from build123d import *

# Parameters (mm, degrees)
SKETCH1_W           = 12
SKETCH1_H           = 12
BOSS_EXTRUDE1_DEPTH = 11
SHELL1_T            = -2
SKETCH3_R           = 0.625
CUT_EXTRUDE1_DEPTH  = 10
SKETCH4_W           = 12
SKETCH4_H           = 12
SKETCH4_W_2         = 11
SKETCH4_H_2         = 11
CUT_EXTRUDE2_DEPTH  = 12
SKETCH5_W           = 11
SKETCH5_H           = 11
CUT_EXTRUDE3_DEPTH  = 0.5


with BuildPart() as part:
    # Sketch1 → Boss-Extrude1 (new body)
    with BuildSketch(Plane(origin=(0, 0, 0), x_dir=(1, 0, 0), z_dir=(0, 1, 0))):
        with Locations((6, 6)):
            Rectangle(SKETCH1_W, SKETCH1_H)
    extrude(amount=BOSS_EXTRUDE1_DEPTH)

    # Shell1
    shell1_openings = [part.faces().sort_by_distance(p)[0] for p in [
        (6, 11, -6),
    ]]
    offset(amount=SHELL1_T, openings=shell1_openings, kind=Kind.INTERSECTION)

    # Sketch3 → Cut-Extrude1 (cut)
    with BuildSketch(Plane.XZ):
        with Locations((6, -4.73)):
            Circle(SKETCH3_R)
        with Locations((6, -7.27)):
            Circle(SKETCH3_R)
    extrude(amount=-CUT_EXTRUDE1_DEPTH, mode=Mode.SUBTRACT)

    # Sketch4 → Cut-Extrude2 (cut, through all)
    with BuildSketch(Plane(origin=(0, 11, 0), x_dir=(1, 0, 0), z_dir=(0, 1, 0))):
        with Locations((6, 6)):
            Rectangle(SKETCH4_W, SKETCH4_H)
        with Locations((6, 6)):
            Rectangle(SKETCH4_W_2, SKETCH4_H_2, mode=Mode.SUBTRACT)
    extrude(amount=-CUT_EXTRUDE2_DEPTH, mode=Mode.SUBTRACT)

    # Sketch5 → Cut-Extrude3 (cut)
    with BuildSketch(Plane.XZ):
        with Locations((6, -6)):
            Rectangle(SKETCH5_W, SKETCH5_H)
    extrude(amount=-CUT_EXTRUDE3_DEPTH, mode=Mode.SUBTRACT)


solid = part.part
Could you check a few things on this model? Use its own coordinates, in mm. A direction names the side the tool comes from. Coordinates: 2 decimals unless noted, no trailing zeros. Write each loop counter-clockwise with the first axis right and the second up, starting at its lowest first coordinate (ties: lowest second). Pieces come first, ordered by that corner, then holes. Notation, with made-up numbers: M 86.5,15 L 124.5,15 A25 cw 124.5,29 Z; hole C 46.25,-12 d6. An arc over 180 degrees is marked long. One line per question, with ' | ' between items.
1) For pin 1 Ø1.6 at (x, z) = (6, -4.73) entering from +Y; pin 2 Ø1.1 at (x, z) = (6, -7.27) entering from +Y, each with a flat end and sliding along its axis, tell me the tip position at first contact or that it passes through.
Checks:
pin 1: y = 2 | pin 2: through
2) Imagine slicing it at C-C, the plane z = -7.27. Write out the boundary of the cut face in (x, y) (3 decimals).
Checks:
outline: M 0.5,0.5 L 5.375,0.5 L 5.375,2 L 2,2 L 2,11 L 0.5,11 Z; M 6.625,0.5 L 11.5,0.5 L 11.5,11 L 10,11 L 10,2 L 6.625,2 Z
3) Imagine slicing it at D-D, the plane x = 9. Write out the boundary of the cut face in (y, z), and give its area (3 significant figures).
Checks:
outline: M 0.5,-11.5 L 11,-11.5 L 11,-10 L 2,-10 L 2,-2 L 11,-2 L 11,-0.5 L 0.5,-0.5 Z | area: 43.5 mm²
4) For faces 1 (the face through (5.92, 1.24, -6.65)), 2 (the face through (6, 6, -2)), which set-ups out of +Z, -Z, +X, -X, +Y, -Y let a thin tool reach every point of the face, with its end or its side?
Checks:
face 1: +Y, -Y | face 2: +Y
5) If we mould it in two halves opening along X, with no side actions, what happens to faces 3 (the face through (6, 6, -0.5)), 4 (the face through (0.5, 6, -6)), 5 (the face through (6, 2, -6))? For each: released by +X, released by -X, zero draft, split by the parting line, or undercut.
Checks:
face 3: zero draft | face 4: released by -X | face 5: undercut
6) Imagine slicing it at A-A, the plane y = 8.25. Write out the boundary of the cut face in (x, z), and give its area (3 significant figures).
Checks:
outline: M 0.5,-11.5 L 11.5,-11.5 L 11.5,-0.5 L 0.5,-0.5 Z; hole M 2,-10 L 10,-10 L 10,-2 L 2,-2 Z | area: 57.0 mm²
7) I need wall thicknesses on probe 1 along Z at (x, y) = (6, 1.35) (3 decimals); probe 2 along Z at (x, y) = (3.5, 9.75); probe 3 along X at (y, z) = (5, -6.5). Which ranges of each line are inside material? Lowest first, please. Write a range as [from, to].
Checks:
probe 1: [-11.5, -7.895], [-6.645, -5.355], [-4.105, -0.5] | probe 2: [-11.5, -10], [-2, -0.5] | probe 3: [0.5, 2], [10, 11.5]
8) Imagine slicing it at B-B, the plane x = 6. Write out the boundary of the cut face in (y, z) (3 decimals).
Checks:
outline: M 0.5,-11.5 L 11,-11.5 L 11,-10 L 2,-10 L 2,-7.895 L 0.5,-7.895 Z; M 0.5,-6.645 L 2,-6.645 L 2,-5.355 L 0.5,-5.355 Z; M 0.5,-4.105 L 2,-4.105 L 2,-2 L 11,-2 L 11,-0.5 L 0.5,-0.5 Z
